Verification items for this drawing (mm, ordinates from the low corner). A direction names the side the tool comes from. Round coordinates to 2 decimals unless told otherwise and drop trailing zeros. Order: outer loops, then holes, each group sorted by start corner. A loop starts at its lowest first (then second) coordinate and runs counter-clockwise, first axis right, second up. Notation, with made-up numbers: (68.5, 89) -> (117.5, 89) arc R8 ccw to (117.5, 103) -> close; hole circle Ø7 at (63, -9). An arc over 180 degrees is marked (long way). Answer in a Markdown table with one row per item. Add a question column.
1. Draft check along Z on the marked faces 3, 4 and 5. Enter one of: +Z half, -Z half, draft (parallel to the pull), parting line (faces both ways), or undercut.
2. Access from +Z, -Z, +X, -X, +Y, -Y to the whole of each face (thin tool, end or side, straight path). Record for the marked faces 1 and 2.
3. Material ranges on L1, parallel to X at y = 22.25, z = 24.5 (1 decimal); L2, parallel to X at y = 6.25, z = 28.5; L3, parallel to Y at x = 31, z = 7, recorded low to high. Write a range as from..to.
4. Depth check by flat-ended pin: P1, Ø10, axis at x = 12, y = 14, coming from the -Z side; P2, Ø12, axis at x = 20, y = 10, coming from the +Z side; P3, Ø1, axis at y = 21.5, z = 23, coming from the -X side. Enter the tip coordinate at first touch or a pass-through.
5. Sectioned sample at A-A, the plane y = 11.25. Record the boundary of the cut face in (x, z), then the cut area to 3 significant figures.
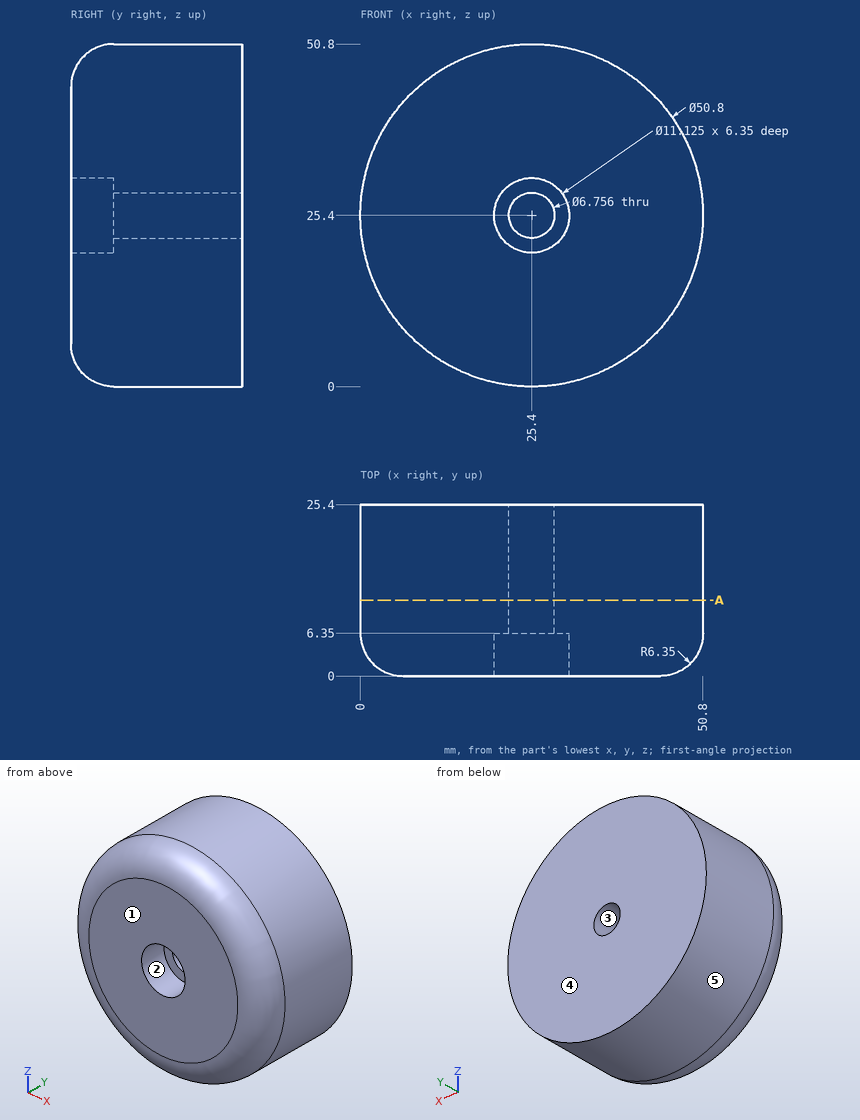
Answer key:
| question | item | result |
|---|---|---|
| 1 | face 3 | undercut |
| 1 | face 4 | draft |
| 1 | face 5 | parting line |
| 2 | face 1 | +Z, -Z, +X, -X, -Y |
| 2 | face 2 | -Y |
| 3 | L1 | x = 0..22.1, 28.7..50.8 |
| 3 | L2 | x = 0.19..20.78, 30.02..50.61 |
| 3 | L3 | y = 0..25.4 |
| 4 | P1 | stops at z = 1.43 |
| 4 | P2 | stops at z = 50.8 |
| 4 | P3 | stops at x = 0.07 |
| 5 | outline | circle Ø50.8 at (25.4, 25.4); hole circle Ø6.76 at (25.4, 25.4) |
| 5 | area | 1,990 mm² |
